Check sheet for the drawn part. Datum: minimum x, y, z corner. Units: mm. A direction names the side the tool comes from. Coordinates: 2 decimals unless noted, no trailing zeros. Loops run counter-clockwise (first coordinate to the right, second up) from the corner with the lowest first, then second, coordinate; pieces in that order, holes last.
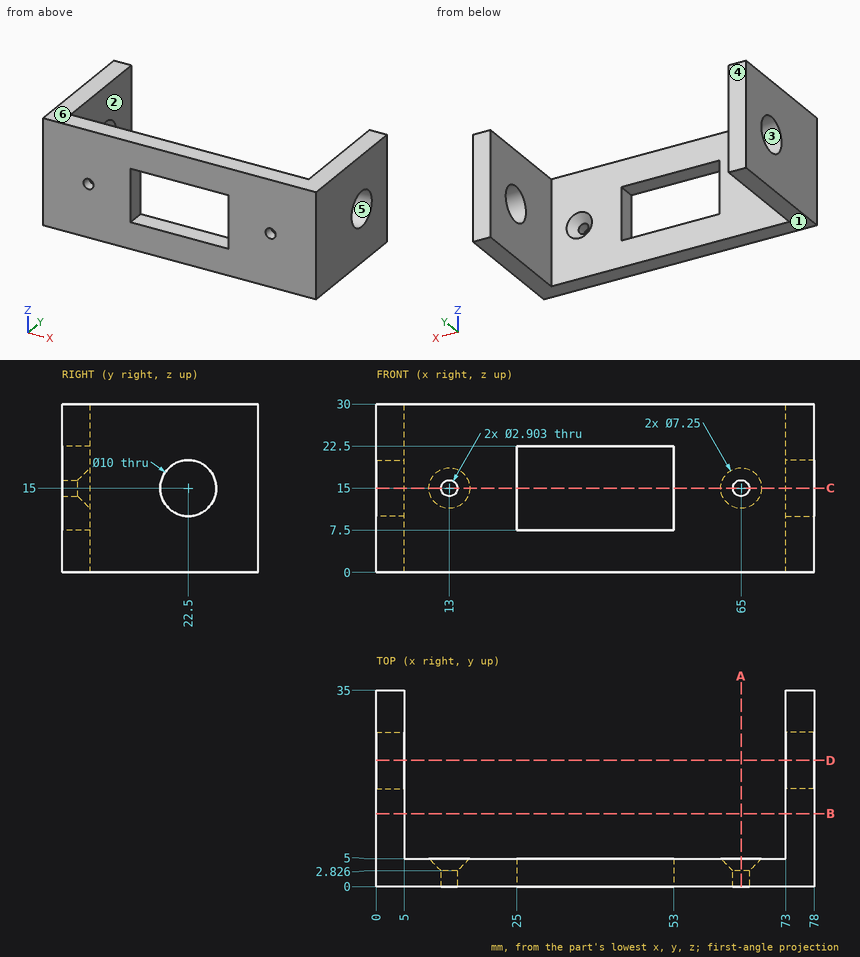
(1) Scan lines: L1, parallel to X at y = 6.5, z = 28; L2, parallel to Y at x = 76.15, z = 15; L3, parallel to Z at x = 74.5, y = 22.5. Record each from-to range of solid material in increasing order.
Findings:
L1: x = 0 to 5, 73 to 78
L2: y = 0 to 17.5, 27.5 to 35
L3: z = 0 to 10, 20 to 30
(2) Sectioned sample at A-A on x = 65. Record the cut outline in (y, z) (1 decimal).
Findings:
outline: (0, 0) - (5, 0) - (5, 11.4) - (2.8, 13.5) - (0, 13.5) - close; (0, 16.5) - (2.8, 16.5) - (5, 18.6) - (5, 30) - (0, 30) - close
(3) Sectioned sample at D-D on y = 22.5. Record the cut outline in (x, z), and give its area (3 significant figures).
Findings:
outline: (0, 0) - (5, 0) - (5, 10) - (0, 10) - close; (0, 20) - (5, 20) - (5, 30) - (0, 30) - close; (73, 0) - (78, 0) - (78, 10) - (73, 10) - close; (73, 20) - (78, 20) - (78, 30) - (73, 30) - close
area: 200 mm2
(4) Access from +Z, -Z, +X, -X, +Y, -Y to the whole of each face (thin tool, end or side, straight path). Record for the marked faces 1 and 2.
Findings:
face 1: -Z, +X, -X, +Y, -Y
face 2: +Z, -Z, +Y
(5) Gauge pin test, flat ends, axial feed: pin 1 Ø15 at (x, z) = (39.5, 20) entering from +Y; pin 2 Ø1.7 at (x, z) = (65, 15) entering from +Y; pin 3 Ø3.5 at (x, z) = (13, 15) entering from +Y (1 decimal). Record the tip position at first contact, or that the pin passes through.
Findings:
pin 1: stops at y = 5
pin 2: passes through
pin 3: stops at y = 3.1
(6) Sectioned sample at B-B on y = 13. Record the cut outline in (x, z), and give its area (3 significant figures).
Findings:
outline: (0, 0) - (5, 0) - (5, 30) - (0, 30) - close; (73, 0) - (78, 0) - (78, 30) - (73, 30) - close
area: 300 mm2
(7) Sectioned sample at C-C on z = 15. State how many separate pieces and enclosed holes the cut face has.
Findings:
separate pieces: 6
enclosed holes: 0
(8) Draft check along Z on the marked faces 3, 4, 5 and 6. Enter one of: +Z half, -Z half, draft (parallel to the pull), parting line (faces both ways), or undercut.
Findings:
face 3: undercut
face 4: draft
face 5: undercut
face 6: +Z half
